```python
from build123d import *

# Parameters (mm, degrees)
SKETCH1_W           = 91.9988
SKETCH1_H           = 25.4
BOSS_EXTRUDE1_DEPTH = 5.9944
SKETCH2_R           = 1.778
CUT_EXTRUDE1_DEPTH  = 6.9944
SKETCH3_W           = 5.9944
SKETCH3_H           = 3.175
CUT_EXTRUDE2_DEPTH  = 6.9944


with BuildPart() as part:
    # Sketch1 → Boss-Extrude1 (new body)
    with BuildSketch(Plane.XY):
        with Locations((45.9994, 12.7)):
            Rectangle(SKETCH1_W, SKETCH1_H)
    extrude(amount=-BOSS_EXTRUDE1_DEPTH)

    # Sketch2 → Cut-Extrude1 (cut, through all)
    with BuildSketch(Plane.XY):
        with Locations((2.9972, 12.7)):
            Circle(SKETCH2_R)
        with Locations((89.0016, 12.7)):
            Circle(SKETCH2_R)
    extrude(amount=-CUT_EXTRUDE1_DEPTH, mode=Mode.SUBTRACT)

    # Sketch3 → Cut-Extrude2 (cut, through all)
    with BuildSketch(Plane.XY):
        with Locations((2.9972, 23.8125)):
            Rectangle(SKETCH3_W, SKETCH3_H)
        with Locations((89.0016, 23.8125)):
            Rectangle(SKETCH3_W, SKETCH3_H)
        with Locations((89.0016, 1.5875)):
            Rectangle(SKETCH3_W, SKETCH3_H)
        with Locations((2.9972, 1.5875)):
            Rectangle(SKETCH3_W, SKETCH3_H)
    extrude(amount=-CUT_EXTRUDE2_DEPTH, mode=Mode.SUBTRACT)


solid = part.part
```
Geometry check sheet. Reference: the model listing, model coordinates, mm. A direction names the side the tool comes from. Round coordinates to 2 decimals unless told otherwise and drop trailing zeros. Loops run counter-clockwise (first coordinate to the right, second up) from the corner with the lowest first, then second, coordinate; pieces in that order, holes last. Notation, with made-up numbers: (-28.5, 43) - (28.5, 43) arc R8 ccw to (28.5, 49) - close; hole circle Ø2 at (27, 26.25). An arc over 180 degrees is marked (long way). Write each question's results on one line, items separated by ' | '. Start each with the question number.
Q1. Gauge pin test, flat ends, axial feed: P1, Ø1, axis at y = 1.5, z = -3, coming from the +X side; P2, Ø1.5, axis at x = 23.5, z = -1, coming from the -Y side. Record the tip position at first contact, or that the pin passes through.
Q2. Cross-section at A-A on y = 12.7. Enter the section's corners in (x, z), and give its area (3 significant figures).
Q3. Cross-section at B-B on z = -2.05. Enter the section's corners in (x, y) (3 decimals).
Q4. Thickness scan on line 1 (X direction, y = 12.5, z = -5.6); line 2 (X direction, y = 12, z = -5.1); line 3 (X direction, y = 23.25, z = -3.75). Record the ranges inside material, lowest first. Write a range as [from, to].
Q5. Release check for a two-part mould opening along Y. For faces 1 (the flat face through (3, 3.175, -3)), 2 (the flat face through (45, 13, -5.994)), 3 (the cylindrical face through (2.766, 14.463, -2.955)) record: +Y half, -Y half, draft (parallel to the pull), parting line (faces both ways), or undercut.
Q6. Access from +Z, -Z, +X, -X, +Y, -Y to the whole of each face (thin tool, end or side, straight path). Record for faces 4 (the flat face through (89, 3.175, -3)), 5 (the flat face through (3, 22.225, -3)), 6 (the flat face through (86.004, 24, -3)), 7 (the flat face through (5.994, 2, -3)).
Answers below:
1) P1: stops at x = 86 | P2: stops at y = 0
2) outline: (0, -5.99) - (1.22, -5.99) - (1.22, 0) - (0, 0) - close; (4.78, -5.99) - (87.22, -5.99) - (87.22, 0) - (4.78, 0) - close; (90.78, -5.99) - (92, -5.99) - (92, 0) - (90.78, 0) - close | area: 509 mm²
3) outline: (0, 3.175) - (5.994, 3.175) - (5.994, 0) - (86.004, 0) - (86.004, 3.175) - (91.999, 3.175) - (91.999, 22.225) - (86.004, 22.225) - (86.004, 25.4) - (5.994, 25.4) - (5.994, 22.225) - (0, 22.225) - close; hole circle Ø3.556 at (2.997, 12.7); hole circle Ø3.556 at (89.002, 12.7)
4) line 1: x = [0, 1.23], [4.76, 87.23], [90.77, 92] | line 2: x = [0, 1.36], [4.63, 87.37], [90.64, 92] | line 3: x = [5.99, 86]
5) face 1: -Y half | face 2: draft | face 3: undercut
6) face 4: +Z, -Z, +X, -Y | face 5: +Z, -Z, -X, +Y | face 6: +Z, -Z, +X, +Y | face 7: +Z, -Z, -X, -Y
